The listing builds one solid part. Answer for the finished solid, in the listing's coordinates (mm). Coordinates: 2 decimals unless noted, no trailing zeros. Loops run counter-clockwise (first coordinate to the right, second up) from the corner with the lowest first, then second, coordinate; pieces in that order, holes last. Notation, with made-up numbers: (87, -9) - (122, -9) arc R24 cw to (122, 18) - close; hole circle Ø6 at (16, 46). An arc over 180 degrees is marked (long way). One line per question, with ' | ' between items.
from build123d import *

# Parameters (mm, degrees)
SKETCH1_W           = 120
SKETCH1_H           = 55
SKETCH1_R           = 1.5
BOSS_EXTRUDE1_DEPTH = 3
CUT_EXTRUDE1_DEPTH  = 67.070038595
SKETCH3_W           = 120
SKETCH3_H           = 3
CUT_EXTRUDE2_DEPTH  = 67.070038595


with BuildPart() as part:
    # Sketch1 → Boss-Extrude1 (new body)
    with BuildSketch(Plane.XY):
        Rectangle(SKETCH1_W, SKETCH1_H)
        with Locations((30, 4.5)):
            Circle(SKETCH1_R, mode=Mode.SUBTRACT)
        with Locations((30, 12.5)):
            Circle(SKETCH1_R, mode=Mode.SUBTRACT)
        with Locations((56, 0)):
            Circle(SKETCH1_R, mode=Mode.SUBTRACT)
        with Locations((48, 0)):
            Circle(SKETCH1_R, mode=Mode.SUBTRACT)
        with Locations((-56, 10)):
            Circle(SKETCH1_R, mode=Mode.SUBTRACT)
        with Locations((-48, 10)):
            Circle(SKETCH1_R, mode=Mode.SUBTRACT)
        with Locations(Location((-56, -10, 0), (0, 0, 180))):
            Circle(SKETCH1_R, mode=Mode.SUBTRACT)
        with Locations(Location((-48, -10, 0), (0, 0, 180))):
            Circle(SKETCH1_R, mode=Mode.SUBTRACT)
        with Locations((-56, 0)):
            Circle(SKETCH1_R, mode=Mode.SUBTRACT)
        with Locations((-48, 0)):
            Circle(SKETCH1_R, mode=Mode.SUBTRACT)
    extrude(amount=BOSS_EXTRUDE1_DEPTH)

    # Sketch2 → Cut-Extrude1 (cut, through all)
    with BuildSketch(Plane.XY.offset(3)):
        Polygon((-60, 15.5), (60, 15.5), (60, 27.5), (-60, 27.514094308), (-60, 27.5), align=None)
    extrude(amount=-CUT_EXTRUDE1_DEPTH, mode=Mode.SUBTRACT)

    # Sketch3 → Cut-Extrude2 (cut, through all)
    with BuildSketch(Plane.XY.offset(3)):
        with Locations((0, -26)):
            Rectangle(SKETCH3_W, SKETCH3_H)
    extrude(amount=-CUT_EXTRUDE2_DEPTH, mode=Mode.SUBTRACT)


solid = part.part
Item 1: Find section C-C, the plane x = 30. Write down the section's boundary in (y, z).
Taken from the geometry:
outline: (-24.5, 0) - (3, 0) - (3, 3) - (-24.5, 3) - close; (6, 0) - (11, 0) - (11, 3) - (6, 3) - close; (14, 0) - (15.5, 0) - (15.5, 3) - (14, 3) - close
Item 2: Find section D-D, the plane x = -48. Write down the section's boundary in (y, z).
Taken from the geometry:
outline: (-24.5, 0) - (-11.5, 0) - (-11.5, 3) - (-24.5, 3) - close; (-8.5, 0) - (-1.5, 0) - (-1.5, 3) - (-8.5, 3) - close; (1.5, 0) - (8.5, 0) - (8.5, 3) - (1.5, 3) - close; (11.5, 0) - (15.5, 0) - (15.5, 3) - (11.5, 3) - close
Item 3: The mould has two halves that part along Y. Classify faces 1 (the face through (57.43, 0.45, 1.48)), 2 (the face through (-1, -24.5, 2)), 3 (the face through (-60, -5, 1)): pulls with the +Y half, pulls with the -Y half, needs draft (parallel to the pull), parting line crosses it, or undercut.
Taken from the geometry:
face 1: undercut | face 2: pulls with the -Y half | face 3: needs draft
Item 4: Find section B-B, the plane y = -10. Write down the section's boundary in (x, z), plus the area to 3 significant figures.
Taken from the geometry:
outline: (-60, 0) - (-57.5, 0) - (-57.5, 3) - (-60, 3) - close; (-54.5, 0) - (-49.5, 0) - (-49.5, 3) - (-54.5, 3) - close; (-46.5, 0) - (60, 0) - (60, 3) - (-46.5, 3) - close | area: 342 mm2
Item 5: Find section A-A, the plane y = 0. Write down the section's boundary in (x, z), plus the area to 3 significant figures.
Taken from the geometry:
outline: (-60, 0) - (-57.5, 0) - (-57.5, 3) - (-60, 3) - close; (-54.5, 0) - (-49.5, 0) - (-49.5, 3) - (-54.5, 3) - close; (-46.5, 0) - (46.5, 0) - (46.5, 3) - (-46.5, 3) - close; (49.5, 0) - (54.5, 0) - (54.5, 3) - (49.5, 3) - close; (57.5, 0) - (60, 0) - (60, 3) - (57.5, 3) - close | area: 324 mm2
Item 6: Find the intervals of material crossed by line 1 (X direction, y = -10, z = 2.3); line 2 (Y direction, x = -56, z = 2); line 3 (X direction, y = 1, z = 2.55), in increasing order. Write a range as [from, to].
Taken from the geometry:
line 1: x = [-60, -57.5], [-54.5, -49.5], [-46.5, 60] | line 2: y = [-24.5, -11.5], [-8.5, -1.5], [1.5, 8.5], [11.5, 15.5] | line 3: x = [-60, -57.12], [-54.88, -49.12], [-46.88, 46.88], [49.12, 54.88], [57.12, 60]
